Autodesk Inventor part; units mm, degrees
ref_plane "YZ Plane" through (0, 0, 0) normal (1, 0, 0) x (0, 1, 0)
ref_plane "XZ Plane" through (0, 0, 0) normal (0, 1, 0) x (-1, 0, 0)
ref_plane "XY Plane" through (0, 0, 0) normal (0, 0, 1) x (1, 0, 0)
sketch "Sketch1" plane through (0, 0, 0) normal (0, 1, 0) x (-1, 0, 0)
  line L0 (27.5, -27.5) -> (-27.5, -27.5)
  line L1 (-27.5, -27.5) -> (-27.5, 27.5)
  line L2 (-27.5, 27.5) -> (27.5, 27.5)
  line L3 (27.5, 27.5) -> (27.5, -27.5)
  line L4 (27.5, 0) -> (-27.5, 0)
  line L5 (0, -27.5) -> (0, 27.5)
  point P0 (0, 0)
  dimension "d3" = 55
  dimension "d4" = 55
extrude "Extrusion1" add sketch "Sketch1" along normal blind 3
chamfer "Chamfer1" distance 5 angle 45 4 edges at (-27.5, 1.5, 27.5) (27.5, 1.5, 27.5) (27.5, 1.5, -27.5) (-27.5, 1.5, -27.5)
sketch "Sketch3" plane through (0, 3, 0) normal (0, 1, 0) x (1, 0, 0)
  line L0 (22.5, 27.5) -> (27.5, 22.5)
  line L1 (25, 25) -> (-25, -25)
  line L2 (-22.5, -27.5) -> (-27.5, -22.5)
  point P0 (0, 0)
  point P1 (7.3223, 7.3223)
  point P2 (21.4645, 21.4645)
  dimension "d12" = 20
  dimension "d13" = 5
hole "Hole1" at (7.3223, 3, -7.3223) at (21.4645, 3, -21.4645) direction (0, -1, 0) diameter 2.3 end through all
mirror "Mirror1" about plane through (0, 0, 0) normal (0, 0, 1) of "Hole1"
mirror "Mirror2" about plane through (0, 0, 0) normal (1, 0, 0) of "Hole1", "Mirror1"
properties part number "Top Plate"
Part model, mm, in its own coordinate system. Coordinates: 2 decimals unless noted, no trailing zeros. Order: outer loops, then holes, each group sorted by start corner. A loop starts at its lowest first (then second) coordinate and runs counter-clockwise, first axis right, second up. Notation, with made-up numbers: M -17.75,72 L 22.25,72 A7 ccw 22.25,81 Z; hole C -36,56.25 d5. An arc over 180 degrees is marked long. One line per question, with ' | ' between items.
Q1. Slice it at C-C (x = 24). Give the cut face in (y, z), and give its area (3 significant figures).
A:
outline: M 0,-26 L 3,-26 L 3,26 L 0,26 Z | area: 156 mm^2
Q2. Slice it at B-B (y = 0.6). Count the separate pieces of the cut face and the enclosed holes in it, and give its area (3 significant figures).
A:
separate pieces: 1 | enclosed holes: 8 | area: 2,940 mm^2
Q3. Two-plate mould, pull along X, no slides. Class faces 1 (the face through (6.88, 1.48, 6.26)), 2 (the face through (0, 1, 27.5)), 3 (the face through (-27.5, 1, 0)): +X half, -X half, draft (parallel to the pull), parting line (faces both ways), or undercut.
A:
face 1: undercut | face 2: draft | face 3: -X half
Q4. Pin check, flat tip, straight feed: P1, Ø1.8, axis at x = 21.46, z = 21.46, coming from the +Y side. Stop position of the tip, or through.
A:
P1: passes through
Q5. Drill centre lines: line 1 (Z direction, x = 21.5, y = 2.25); line 2 (Z direction, x = 21, y = 0.55). Where is each one in solid material? Low to high.
A:
line 1: z = -27.5 to -22.61, -20.32 to 20.32, 22.61 to 27.5 | line 2: z = -27.5 to -22.52, -20.41 to 20.41, 22.52 to 27.5
Q6. Slice it at A-A (z = 21.5). Give the cut face in (x, y).
A:
outline: M -27.5,0 L -22.61,0 L -22.61,3 L -27.5,3 Z; M -20.32,0 L 20.32,0 L 20.32,3 L -20.32,3 Z; M 22.61,0 L 27.5,0 L 27.5,3 L 22.61,3 Z
